Source: CAD feature listing. Evaluate the final solid. Frame: model axes, mm. Round coordinates to 2 decimals unless told otherwise and drop trailing zeros. Write each loop counter-clockwise with the first axis right and the second up, starting at its lowest first coordinate (ties: lowest second). Pieces come first, ordered by that corner, then holes.
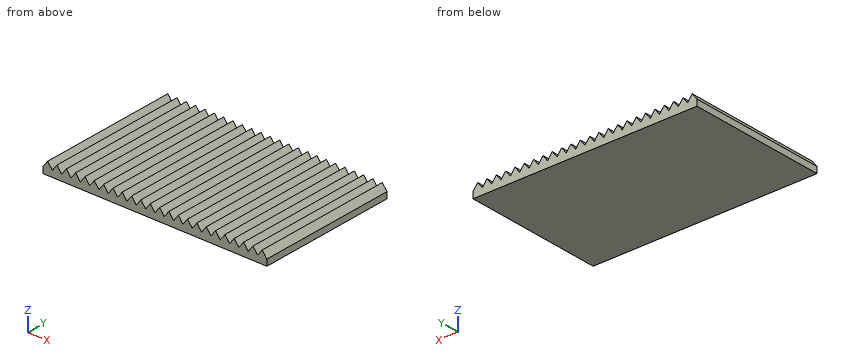
```python
from build123d import *

# Parameters (mm, degrees)
F1_DEPTH = 254


# Not quite as in the source:
# - ends of sketch curves that miss each other by under 0.0002 mm in the source are joined


with BuildPart() as f1:
    # F0 (on Front) → F1 (new body)
    with BuildSketch(Plane.XZ):
        Polygon((-194.73333335, 16.9333332013), (-203.2, 5.6444444388), (-194.73333335, 5.6444444388), align=None)
        Polygon((-194.73333335, 5.6444444388), (-203.2, 5.6444444388), (-203.2, -5.6444444388), (203.2, -5.6444444388), (203.2, 5.6444444388), (186.26665915, 5.6444444388), (169.33332615, 5.6444444388), (152.39999315, 5.6444444388), (135.46666015, 5.6444444388), (118.53332715, 5.6444444388), (101.59999415, 5.6444444388), (84.66666115, 5.6444444388), (67.73332815, 5.6444444388), (50.79999515, 5.6444444388), (33.86666215, 5.6444444388), (16.93332915, 5.6444444388), (-3.85e-06, 5.6444444388), (-16.93333685, 5.6444444388), (-33.86666985, 5.6444444388), (-50.80000285, 5.6444444388), (-67.73333585, 5.6444444388), (-84.66666885, 5.6444444388), (-101.60000185, 5.6444444388), (-118.53333485, 5.6444444388), (-135.46666785, 5.6444444388), (-152.40000085, 5.6444444388), (-169.33333385, 5.6444444388), (-186.26666685, 5.6444444388), align=None)
        Polygon((-194.73333335, 16.9333332013), (-194.73333335, 5.6444444388), (-186.26666685, 5.6444444388), align=None)
        Polygon((-177.80000035, 16.9333332013), (-186.266667, 5.6444444388), (-169.33333385, 5.6444444388), align=None)
        Polygon((-160.86666735, 16.9333332013), (-169.333334, 5.6444444388), (-152.40000085, 5.6444444388), align=None)
        Polygon((186.26665915, 5.6444444388), (203.2, 5.6444444388), (194.73332565, 16.9333332013), align=None)
        Polygon((-143.93333435, 16.9333332013), (-152.400001, 5.6444444388), (-135.46666785, 5.6444444388), align=None)
        Polygon((169.33332615, 5.6444444388), (186.26665915, 5.6444444388), (177.79999265, 16.9333332013), align=None)
        Polygon((-127.00000135, 16.9333332013), (-135.466668, 5.6444444388), (-118.53333485, 5.6444444388), align=None)
        Polygon((152.39999315, 5.6444444388), (169.33332615, 5.6444444388), (160.86665965, 16.9333332013), align=None)
        Polygon((-110.06666835, 16.9333332013), (-118.533335, 5.6444444388), (-101.60000185, 5.6444444388), align=None)
        Polygon((135.46666015, 5.6444444388), (152.39999315, 5.6444444388), (143.93332665, 16.9333332013), align=None)
        Polygon((-93.13333535, 16.9333332013), (-101.600002, 5.6444444388), (-84.66666885, 5.6444444388), align=None)
        Polygon((118.53332715, 5.6444444388), (135.46666015, 5.6444444388), (126.99999365, 16.9333332013), align=None)
        Polygon((-76.20000235, 16.9333332013), (-84.666669, 5.6444444388), (-67.73333585, 5.6444444388), align=None)
        Polygon((101.59999415, 5.6444444388), (118.53332715, 5.6444444388), (110.06666065, 16.9333332013), align=None)
        Polygon((-59.26666935, 16.9333332013), (-67.733336, 5.6444444388), (-50.80000285, 5.6444444388), align=None)
        Polygon((84.66666115, 5.6444444388), (101.59999415, 5.6444444388), (93.13332765, 16.9333332013), align=None)
        Polygon((-42.33333635, 16.9333332013), (-50.800003, 5.6444444388), (-33.86666985, 5.6444444388), align=None)
        Polygon((67.73332815, 5.6444444388), (84.66666115, 5.6444444388), (76.19999465, 16.9333332013), align=None)
        Polygon((-25.40000335, 16.9333332013), (-33.86667, 5.6444444388), (-16.93333685, 5.6444444388), align=None)
        Polygon((50.79999515, 5.6444444388), (67.73332815, 5.6444444388), (59.26666165, 16.9333332013), align=None)
        Polygon((-8.46667035, 16.9333332013), (-16.933337, 5.6444444388), (-3.85e-06, 5.6444444388), align=None)
        Polygon((33.86666215, 5.6444444388), (50.79999515, 5.6444444388), (42.33332865, 16.9333332013), align=None)
        Polygon((8.46666265, 16.9333332013), (-4e-06, 5.6444444388), (16.93332915, 5.6444444388), align=None)
        Polygon((16.93332915, 5.6444444388), (33.86666215, 5.6444444388), (25.39999565, 16.9333332013), align=None)
    extrude(amount=F1_DEPTH)


solid = f1.part
```
Q1. Line query: line 1 (Z direction, x = 10, y = -187.5); line 2 (Z direction, x = 165.5, y = -126.5). Output: solid intervals per line, ascending.
Q2. Section query A-A, the plane z = 11. Give the number of separate pieces and of enclosed holes in the cut face, and give its area (3 significant figures).
Q3. Pin query (flat end, axial travel): P1, Ø6, axis at x = 112, z = 7, coming from the +Y side; P2, Ø12, axis at x = -68, y = -89.5, coming from the +Z side; P3, Ø8, axis at x = 54, y = -153, coming from the +Z side. Return the tip coordinate at first contact, or that it passes through.
Q4. Section query B-B, the plane x = 4. Output: boundary loops of the cut face in (y, z), and give its area (3 significant figures).
Filled in:
1. line 1: z = -5.64 to 14.89
1. line 2: z = -5.64 to 10.76
2. separate pieces: 24
2. enclosed holes: 0
2. area: 54,300 mm2
3. P1: stops at y = 0
3. P2: stops at z = 14
3. P3: stops at z = 15.24
4. outline: (-254, -5.64) - (0, -5.64) - (0, 10.98) - (-254, 10.98) - close
4. area: 4,220 mm2
